Check sheet for the modelled part. Datum: model origin and axes. Units: mm. Coordinates: 2 decimals unless noted, no trailing zeros. Write each loop counter-clockwise with the first axis right and the second up, starting at its lowest first coordinate (ties: lowest second). Pieces come first, ordered by that corner, then holes. Notation, with made-up numbers: (63.5, -5) - (89.5, -5) arc R26 ccw to (89.5, 21) - close; hole circle Ø6 at (40.5, 58.5). An arc over 180 degrees is marked (long way). Use one line per item in the form item = value. Start each with the question number.
1. Scan lines: line 1 along Y through (x, z) = (0, 5); line 2 along Z through (x, y) = (-12.5, 34); line 3 along Y through (x, z) = (1, 8.5). Record each from-to range of solid material in increasing order.
2. Cross-section at A-A on z = 25.5. Record the boundary of the cut face in (x, y), then the cut area to 3 significant figures.
3. Cross-section at C-C on z = 20. Record the boundary of the cut face in (x, y), then the cut area to 3 significant figures.
4. Cross-section at B-B on z = 11.5. Record the boundary of the cut face in (x, y), then the cut area to 3 significant figures.
5. Go/stop test with flat-tipped pins: pin 1 Ø1.8 at (x, y) = (10, 20.5) entering from +Z; pin 2 Ø5 at (x, z) = (7.5, 19) entering from +Y; pin 3 Ø2 at (y, z) = (39, 0.5) entering from +X; pin 4 Ø4 at (x, y) = (10, 30.5) entering from +Z. Record where each tip stops, or that it passes through.
```python
from build123d import *

# Parameters (mm, degrees)
BOSS_EXTRUDE1_DEPTH = 10
FILLET1_R           = 5
FILLET2_R           = 5
FILLET3_R           = 2
FILLET4_R           = 2
FILLET5_R           = 5
FILLET6_R           = 5
FILLET7_R           = 2
FILLET8_R           = 2
SKETCH2_R           = 7.5
BOSS_EXTRUDE2_DEPTH = 20
CUT_EXTRUDE1_DEPTH  = 57.781501862
SKETCH5_R           = 2.5
CUT_EXTRUDE3_DEPTH  = 57.781501914
SKETCH11_R          = 1.5
CUT_EXTRUDE6_DEPTH  = 57.781501914
SKETCH12_R          = 1.5
CUT_EXTRUDE7_DEPTH  = 57.781501914


with BuildPart() as part:
    # Sketch1 → Boss-Extrude1 (new body)
    with BuildSketch(Plane.XY):
        Polygon((0, 0), (10, 0), (30, 40), (0, 40), align=None)
    boss_extrude1 = extrude(amount=BOSS_EXTRUDE1_DEPTH)

    # Fillet1
    fillet1_edges = [part.edges().sort_by_distance(p)[0] for p in [
        (30, 40, 5),
    ]]
    fillet(fillet1_edges, radius=FILLET1_R)

    # Fillet2
    fillet2_edges = [part.edges().sort_by_distance(p)[0] for p in [
        (10, 0, 5),
    ]]
    fillet(fillet2_edges, radius=FILLET2_R)

    # Fillet3
    fillet3_edges = [part.edges().sort_by_distance(p)[0] for p in [
        (10.954915028, 40, 10),
        (26.163084098, 37.628655561, 10),
        (18.881966011, 17.763932023, 10),
        (9.538485617, 0.746745958, 10),
        (3.454915028, 0, 10),
    ]]
    fillet(fillet3_edges, radius=FILLET3_R)

    # Fillet4
    fillet4_edges = [part.edges().sort_by_distance(p)[0] for p in [
        (10.954915028, 40, 0),
        (26.163084098, 37.628655561, 0),
        (18.881966011, 17.763932023, 0),
        (9.538485617, 0.746745958, 0),
        (3.454915028, 0, 0),
    ]]
    fillet(fillet4_edges, radius=FILLET4_R)

    # Mirror1: Boss-Extrude1 across plane
    add(boss_extrude1.mirror(Plane(origin=(0, 0, 0), x_dir=(0, 0, 1), z_dir=(1, 0, 0))))

    # Fillet5
    fillet5_edges = [part.edges().sort_by_distance(p)[0] for p in [
        (-30, 40, 5),
    ]]
    fillet(fillet5_edges, radius=FILLET5_R)

    # Fillet6
    fillet6_edges = [part.edges().sort_by_distance(p)[0] for p in [
        (-10, 0, 5),
    ]]
    fillet(fillet6_edges, radius=FILLET6_R)

    # Fillet7
    fillet7_edges = [part.edges().sort_by_distance(p)[0] for p in [
        (-3.454915028, 0, 0),
        (-9.538485617, 0.746745958, 0),
        (-10.954915028, 40, 0),
        (-26.163084098, 37.628655561, 0),
        (-18.881966011, 17.763932023, 0),
    ]]
    fillet(fillet7_edges, radius=FILLET7_R)

    # Fillet8
    fillet8_edges = [part.edges().sort_by_distance(p)[0] for p in [
        (-3.454915028, 0, 10),
        (-9.538485617, 0.746745958, 10),
        (-10.954915028, 40, 10),
        (-26.163084098, 37.628655561, 10),
        (-18.881966011, 17.763932023, 10),
    ]]
    fillet(fillet8_edges, radius=FILLET8_R)

    # Sketch2 → Boss-Extrude2 (add)
    with BuildSketch(Plane.XY.offset(10)):
        with Locations((0, 10)):
            Circle(SKETCH2_R)
    extrude(amount=BOSS_EXTRUDE2_DEPTH)

    # Sketch4 → Cut-Extrude1 (cut, through all)
    with BuildSketch(Plane(origin=(0, 0, 0), x_dir=(0, 0, -1), z_dir=(1, 0, 0))):
        with BuildLine():
            Line((-21.5, 12.5), (-30, 12.5))
            Line((-30, 12.5), (-30, 7.5))
            Line((-30, 7.5), (-21.5, 7.5))
            ThreePointArc((-21.5, 7.5), (-19, 10), (-21.5, 12.5))
        make_face()
    cut_extrude1 = extrude(amount=-CUT_EXTRUDE1_DEPTH, mode=Mode.SUBTRACT)

    # Mirror2: Cut-Extrude1 across plane
    add(cut_extrude1.mirror(Plane(origin=(0, 0, 0), x_dir=(0, 0, 1), z_dir=(1, 0, 0))), mode=Mode.SUBTRACT)

    # Sketch5 → Cut-Extrude3 (cut, through all)
    with BuildSketch(Plane(origin=(0, 0, 0), x_dir=(1, 0, 0), z_dir=(0, 1, 0))):
        with Locations(Location((0, -25, 0), (0, 0, 90))):
            Circle(SKETCH5_R)
    extrude(amount=CUT_EXTRUDE3_DEPTH, mode=Mode.SUBTRACT)

    # Sketch11 → Cut-Extrude6 (cut, through all)
    with BuildSketch(Plane(origin=(0, 0, 0), x_dir=(-1, 0, 0), z_dir=(0, 0, -1))):
        with Locations((0, 30.50121957)):
            Circle(SKETCH11_R)
        with Locations((-10, 30.50121957)):
            Circle(SKETCH11_R)
        with Locations((10, 30.50121957)):
            Circle(SKETCH11_R)
        with Locations((0, 20.50121957)):
            Circle(SKETCH11_R)
        with Locations((10, 20.50121957)):
            Circle(SKETCH11_R)
        with Locations((-10, 20.50121957)):
            Circle(SKETCH11_R)
    extrude(amount=-CUT_EXTRUDE6_DEPTH, mode=Mode.SUBTRACT)

    # Sketch12 → Cut-Extrude7 (cut, through all)
    with BuildSketch(Plane(origin=(0, 0, 0), x_dir=(0, 0, -1), z_dir=(1, 0, 0))):
        with Locations((-5, 34)):
            Circle(SKETCH12_R)
    cut_extrude7 = extrude(amount=-CUT_EXTRUDE7_DEPTH, mode=Mode.SUBTRACT)

    # Mirror3: Cut-Extrude7 across plane
    add(cut_extrude7.mirror(Plane(origin=(0, 0, 0), x_dir=(0, 0, 1), z_dir=(1, 0, 0))), mode=Mode.SUBTRACT)


solid = part.part
```
Final values:
q1.line_1 = 0 to 19, 22 to 29, 32 to 32.5, 35.5 to 40
q1.line_2 = 0 to 3.5, 6.5 to 10
q1.line_3 = 0.06 to 19.38, 21.62 to 29.38, 31.62 to 39.94
q2.outline = (-7.07, 7.5) arc R7.5 ccw to (-2.45, 2.91) - (-2.45, 7.5) - close; (-7.07, 12.5) - (-2.45, 12.5) - (-2.45, 17.09) arc R7.5 ccw to start; (2.45, 2.91) arc R7.5 ccw to (7.07, 7.5) - (2.45, 7.5) - close; (2.45, 12.5) - (7.07, 12.5) arc R7.5 ccw to (2.45, 17.09) - close
q2.area = 55.5 mm²
q3.outline = (-7.23, 8) arc R7.5 ccw to (7.23, 8) - close; (-7.23, 12) - (7.23, 12) arc R7.5 ccw to start
q3.area = 117 mm²
q4.outline = circle Ø15 at (0, 10)
q4.area = 177 mm²
q5.pin_1 = through
q5.pin_2 = 15.59
q5.pin_3 = 25.47
q5.pin_4 = 10
